Autodesk Inventor part; units mm, degrees
ref_plane "YZ Plane" through (0, 0, 0) normal (1, 0, 0) x (0, 1, 0)
ref_plane "XZ Plane" through (0, 0, 0) normal (0, 1, 0) x (-1, 0, 0)
ref_plane "XY Plane" through (0, 0, 0) normal (0, 0, 1) x (1, 0, 0)
sketch "Sketch3" plane through (0, 0, 0) normal (0, 0, 1) x (1, 0, 0)
  circle A0 centre (0, 0) radius 4
  circle A1 centre (0, 0) radius 17.5
  dimension "d0" = 8
  dimension "d1" = 35
extrude "Extrusion1" add sketch "Sketch3" along normal blind 5
sketch "Sketch4" plane through (0, 0, 5) normal (0, 0, 1) x (1, 0, 0)
  circle A0 centre (0, 0) radius 4
  circle A1 centre (0, 0) radius 8
  dimension "d4" = 16
  dimension "d5" = 8
extrude "Extrusion2" add sketch "Sketch4" along normal blind 55
sketch "Sketch5" plane through (0, 0, 0) normal (0, 0, -1) x (-1, 0, 0)
  circle A0 centre (15, 0) radius 2
  circle A1 centre (0, 15) radius 2
  circle A2 centre (0, -15) radius 2
  circle A3 centre (-15, 0) radius 2
  point P0 (0, 0)
  dimension "d8" = 4
  dimension "d9" = 15
  dimension "d10" = 15
  dimension "d11" = 15
  dimension "d12" = 15
  dimension "d13" = 4
  dimension "d14" = 4
  dimension "d15" = 4
extrude "Extrusion3" cut sketch "Sketch5" against normal through all
equation "\"d0\" = RodDiameter"
equation "\"d4\" = VerticalBearingOD"
equation "\"d5\" = RodDiameter"
equation "\"d13\" = d8"
equation "\"d14\" = d8"
equation "\"d15\" = d8"
equation "\"RodDiameter\" = 8"
equation "\"VerticalBearingOD\" = 16"
equation "\"PrintingClearance\" = 0.2"
properties part number "VerticalBearing"
Read the model definition and answer for the solid it produces. Units are mm, in the model's axes. A direction names the side the tool comes from. Round coordinates to 2 decimals unless told otherwise and drop trailing zeros. Order: outer loops, then holes, each group sorted by start corner. A loop starts at its lowest first (then second) coordinate and runs counter-clockwise, first axis right, second up.
1) The mould has two halves that part along X. Classify faces 3 (the face through (-4, -2, 60)), 4 (the face through (-13.887, 10.648, 2.465)), 5 (the face through (0, -13, 2)): released by +X, released by -X, zero draft, split by the parting line, or undercut.
2) For faces 1 (the face through (-13.4, -1.2, 2.5)), 2 (the face through (-1.73, 7.81, 32.11)), determine the directions among +Z, -Z, +X, -X, +Y, -Y from which every point of the face is accessible in a straight line to the end or side of a thin tool.
3) The part is cut by section B-B on z = 51.5. Write down the section's boundary in (x, y), plus the area to 3 significant figures.
4) Flat-ended cylindrical pins translate along their axes: pin 1 (3.5 mm diameter, centred on x = 0, y = 15, fed in from -Z); pin 2 (6 mm diameter, centred on y = -2, z = 23, fed in from -X); pin 3 (1.5 mm diameter, centred on x = 1.5, z = 34, fed in from +Y); pin 4 (8 mm diameter, centred on y = 0.5, z = 54, fed in from +X). Find the tip coordinate at first contact, or state that the pin passes through.
5) The part is cut by section C-C on x = -15. Write down the section's boundary in (y, z), plus the area to 3 significant figures.
6) Straight lines are drawn through the part: L1, parallel to Z at x = 12, y = -1.5; L2, parallel to Y at x = 0, z = 24.5; L3, parallel to Y at x = 15, z = 4.05. For each, find the intervals that lie inside material, in ascending order.
7) The part is cut by section A-A on y = 0. Write down the section's boundary in (x, z).
Resolved:
1. face 3: zero draft
1. face 4: split by the parting line
1. face 5: undercut
2. face 1: +Z, -Z
2. face 2: +Z
3. outline: circle Ø16 at (0, 0); hole circle Ø8 at (0, 0)
3. area: 151 mm2
4. pin 1: passes through
4. pin 2: stops at x = -8
4. pin 3: stops at y = 7.96
4. pin 4: stops at x = 8
5. outline: (-9.01, 0) - (-2, 0) - (-2, 5) - (-9.01, 5) - close; (2, 0) - (9.01, 0) - (9.01, 5) - (2, 5) - close
5. area: 70.1 mm2
6. L1: z = 0 to 5
6. L2: y = -8 to -4, 4 to 8
6. L3: y = -9.01 to -2, 2 to 9.01
7. outline: (-17.5, 0) - (-17, 0) - (-17, 5) - (-17.5, 5) - close; (-13, 0) - (-4, 0) - (-4, 60) - (-8, 60) - (-8, 5) - (-13, 5) - close; (4, 0) - (13, 0) - (13, 5) - (8, 5) - (8, 60) - (4, 60) - close; (17, 0) - (17.5, 0) - (17.5, 5) - (17, 5) - close
